Check sheet for the modelled part. Datum: model origin and axes. Units: mm. A direction names the side the tool comes from. Round coordinates to 2 decimals unless told otherwise and drop trailing zeros. Write each loop counter-clockwise with the first axis right and the second up, starting at its lowest first coordinate (ties: lowest second). Pieces come first, ordered by that corner, then holes. Notation, with made-up numbers: M 74.25,11 L 110.25,11 A16 cw 110.25,39 Z; hole C -14.5,-19.5 d3. An arc over 180 degrees is marked long. Answer in a Markdown table with one row per item.
```python
from build123d import *

# Parameters (mm, degrees)
SKETCH_1_W      = 300
SKETCH_1_H      = 400
EXTRUDE_1_DEPTH = 10
EXTRUDE_2_DEPTH = 32


with BuildPart() as part:
    # 草图1 → 凸台-拉伸1 (new body)
    with BuildSketch(Plane.XY):
        with Locations((115.046975242, -172.111948332)):
            Rectangle(SKETCH_1_W, SKETCH_1_H)
    extrude(amount=EXTRUDE_1_DEPTH)

    # 草图2 → 凸台-拉伸2 (add)
    with BuildSketch(Plane.XY.offset(10)):
        Polygon((265.046975242, -372.111948332), (265.046975242, 27.888051668), (-34.953024758, 27.888051668), (-34.953024758, -372.111948332), (-24.953024758, -372.111948332), (-24.953024758, 17.888051668), (255.046975242, 17.888051668), (255.046975242, -372.111948332), align=None)
    extrude(amount=EXTRUDE_2_DEPTH)


solid = part.part
```
1. Go/stop test with a flat-tipped pin: pin 1 (9.5 mm diameter, centred on x = 104, z = 27, fed in from -Y). Record where the tip stops, or that it passes through.
Found:
| item | result |
|---|---|
| pin 1 | stops at y = 17.89 |
2. Draft check along X on faces 1 (the face through (-34.953, -169, 21)), 2 (the face through (-24.953, -180, 26)), 3 (the face through (113, -169, 0)). Enter one of: +X half, -X half, draft (parallel to the pull), parting line (faces both ways), or undercut.
Found:
| item | result |
|---|---|
| face 1 | -X half |
| face 2 | undercut |
| face 3 | draft |
3. Scan lines: L1, parallel to X at y = -111, z = 18; L2, parallel to Z at x = 81, y = -94.5; L3, parallel to Y at x = 166, z = 40.5. Record each from-to range of solid material in increasing order.
Found:
| item | result |
|---|---|
| L1 | x = -34.95 to -24.95, 255.05 to 265.05 |
| L2 | z = 0 to 10 |
| L3 | y = 17.89 to 27.89 |
4. Access from +Z, -Z, +X, -X, +Y, -Y to the whole of each face (thin tool, end or side, straight path). Record for faces 4 (the face through (113, 17.888, 26)), 5 (the face through (114, -372.112, 7)).
Found:
| item | result |
|---|---|
| face 4 | +Z, -Y |
| face 5 | +Z, -Z, +X, -X, -Y |
5. Section check C-C, the plane x = 215.5. Record the cut outline in (y, z).
Found:
| item | result |
|---|---|
| outline | M -372.11,0 L 27.89,0 L 27.89,42 L 17.89,42 L 17.89,10 L -372.11,10 Z |
6. Section check A-A, the plane y = -247. Record the cut outline in (x, z), and give its area (3 significant figures).
Found:
| item | result |
|---|---|
| outline | M -34.95,0 L 265.05,0 L 265.05,42 L 255.05,42 L 255.05,10 L -24.95,10 L -24.95,42 L -34.95,42 Z |
| area | 3,640 mm2 |
7. Section check B-B, the plane z = 33.5. Record the cut outline in (x, y), and give its area (3 significant figures).
Found:
| item | result |
|---|---|
| outline | M -34.95,-372.11 L -24.95,-372.11 L -24.95,17.89 L 255.05,17.89 L 255.05,-372.11 L 265.05,-372.11 L 265.05,27.89 L -34.95,27.89 Z |
| area | 10,800 mm2 |
